For this review, use the dimensioned drawing (mm, ordinates from the lowest corner) and the shaded views. A direction names the side the tool comes from. Give positions to 0.01 mm unless a question says otherwise; leave off trailing zeros. Order: outer loops, then holes, each group sorted by start corner. A loop starts at its lowest first (then second) coordinate and runs counter-clockwise, first axis right, second up. Notation, with made-up numbers: (17, -31) - (25, -31) arc R26 ccw to (25, 3) - close; hole circle Ø11 at (33.5, 76). An arc over 180 degrees is marked (long way). Use a Markdown table: item, result. Add a question column.
1) We need section D-D on x = 77. Write out the cut boundary in (y, z).
2) We need section B-B on z = 9.75. Write out the cut boundary in (x, y).
3) Clearance check with flat-ended pins moving along their axes: P1, Ø3, axis at y = 3.5, z = 6, coming from the -X side; P2, Ø4, axis at x = 51, z = 3.5, coming from the -Y side; P3, Ø2.5, axis at x = 32, y = 8, coming from the +Z side; P4, Ø6.5, axis at x = 76.5, z = 9.5, coming from the +Y side. State where each tip first meets the part, or that it passes through.
4) We need section C-C on y = 3. Write out the cut boundary in (x, z), then the cut area to 3 significant figures.
5) Machinability: for the marked faces 1, 2 and 3, which of the approach directions +Z, -Z, +X, -X, +Y, -Y give a long, thin tool a straight path to every point of the face, cutting with its end or side? Answer none if there is none.
6) Wall thickness on L1, parallel to X at y = 3, z = 6; L2, parallel to X at y = 1, z = 1; L3, parallel to Z at x = 2.05, y = 3: over which ranges is each line inside the solid? List them lowest first.
7) We need section A-A on z = 6.5. Write out the cut boundary in (x, y), then the cut area to 3 significant figures.
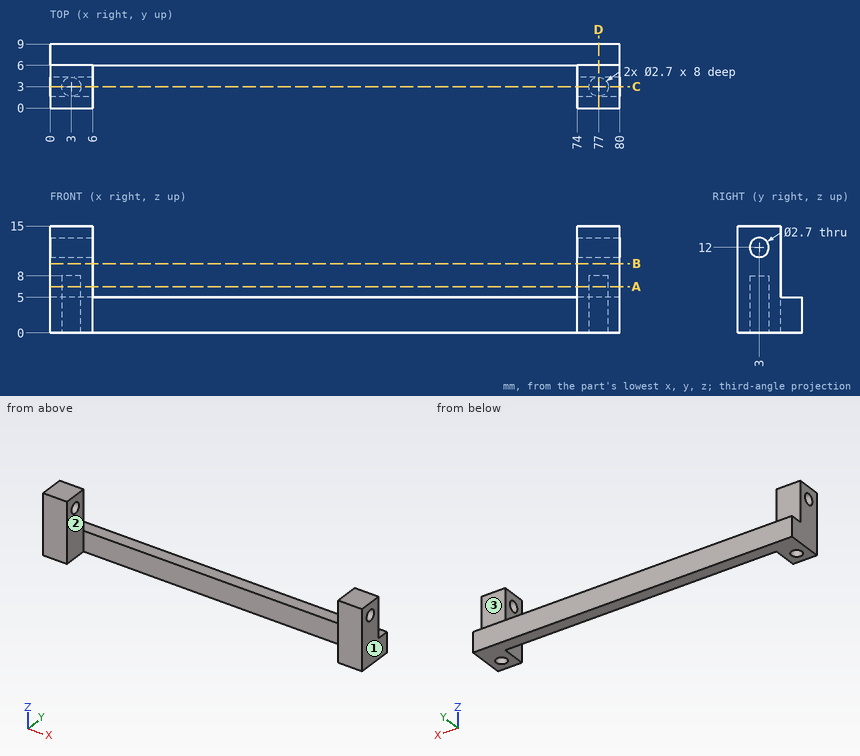
Checked values:
| question | item | result |
|---|---|---|
| 1 | outline | (0, 0) - (1.65, 0) - (1.65, 8) - (4.35, 8) - (4.35, 0) - (9, 0) - (9, 5) - (6, 5) - (6, 15) - (0, 15) - close; hole circle Ø2.7 at (3, 12) |
| 2 | outline | (0, 0) - (6, 0) - (6, 6) - (0, 6) - close; (74, 0) - (80, 0) - (80, 6) - (74, 6) - close |
| 3 | P1 | x = 0 |
| 3 | P2 | y = 6 |
| 3 | P3 | z = 5 |
| 3 | P4 | y = 6 |
| 4 | outline | (0, 0) - (1.65, 0) - (1.65, 8) - (4.35, 8) - (4.35, 0) - (6, 0) - (6, 10.65) - (0, 10.65) - close; (0, 13.35) - (6, 13.35) - (6, 15) - (0, 15) - close; (74, 0) - (75.65, 0) - (75.65, 8) - (78.35, 8) - (78.35, 0) - (80, 0) - (80, 10.65) - (74, 10.65) - close; (74, 13.35) - (80, 13.35) - (80, 15) - (74, 15) - close |
| 4 | area | 104 mm² |
| 5 | face 1 | +Z, -Z, +X, +Y, -Y |
| 5 | face 2 | +Z, -Z, -Y |
| 5 | face 3 | +Z, +X, -X, +Y |
| 6 | L1 | 0 to 1.65, 4.35 to 6, 74 to 75.65, 78.35 to 80 |
| 6 | L2 | 0 to 6, 74 to 80 |
| 6 | L3 | 8 to 10.65, 13.35 to 15 |
| 7 | outline | (0, 0) - (6, 0) - (6, 6) - (0, 6) - close; (74, 0) - (80, 0) - (80, 6) - (74, 6) - close; hole circle Ø2.7 at (3, 3); hole circle Ø2.7 at (77, 3) |
| 7 | area | 60.5 mm² |
